```python
from build123d import *

# Parameters (mm, degrees)
SKETCH1_W           = 44.45
SKETCH1_H           = 50.8
BOSS_EXTRUDE1_DEPTH = 6.35
SKETCH2_W           = 5.08
SKETCH2_H           = 50.8
BOSS_EXTRUDE2_DEPTH = 25.4
SKETCH3_W           = 5.08
SKETCH3_H           = 50.8
BOSS_EXTRUDE3_DEPTH = 19.05
CUT_EXTRUDE1_REACH  = 55.295
CUT_EXTRUDE2_REACH  = 55.295
SKETCH5_R           = 1.905
LPATTERN1_COUNT     = 2
LPATTERN1_PITCH     = 12.7
LPATTERN1_COL_COUNT = 2
LPATTERN1_COL_PITCH = 12.7
CHAMFER3_SIZE       = 5.028946
CHAMFER1_SIZE       = 3.175
CUT_EXTRUDE3_REACH  = 40.756
SKETCH6_W           = 34.392108
SKETCH6_H           = 5.08
LPATTERN2_COUNT     = 2
LPATTERN2_PITCH     = 15.24
LPATTERN2_COL_COUNT = 2
LPATTERN2_COL_PITCH = 15.24
CHAMFER4_SIZE       = 1.27


with BuildPart() as part:
    # Sketch1 → Boss-Extrude1 (new body)
    with BuildSketch(Plane(origin=(0, 0, 0), x_dir=(1, 0, 0), z_dir=(0, 1, 0))):
        Rectangle(SKETCH1_W, SKETCH1_H)
    extrude(amount=BOSS_EXTRUDE1_DEPTH)

    # Sketch2 → Boss-Extrude2 (add)
    with BuildSketch(Plane(origin=(0, 0, 0), x_dir=(1, 0, 0), z_dir=(0, 1, 0))):
        with Locations((-19.685, 0)):
            Rectangle(SKETCH2_W, SKETCH2_H)
    extrude(amount=BOSS_EXTRUDE2_DEPTH)

    # Sketch3 → Boss-Extrude3 (add)
    with BuildSketch(Plane(origin=(0, 0, 0), x_dir=(1, 0, 0), z_dir=(0, 1, 0))):
        with Locations((19.685, 0)):
            Rectangle(SKETCH3_W, SKETCH3_H)
    extrude(amount=BOSS_EXTRUDE3_DEPTH)

    # Sketch4 → Cut-Extrude1 (cut, up to next)
    with BuildSketch(Plane(origin=(-17.145, 0, 0), x_dir=(0, 0, -1), z_dir=(1, 0, 0)), mode=Mode.PRIVATE) as cut_extrude1_sk1:
        with BuildLine():
            Line((-2.38125, 11.90625), (-2.38125, 19.84375))
            ThreePointArc((-2.38125, 19.84375), (0, 22.225), (2.38125, 19.84375))
            Line((2.38125, 19.84375), (2.38125, 11.90625))
            ThreePointArc((2.38125, 11.90625), (0, 9.525), (-2.38125, 11.90625))
        make_face()
    cut_extrude1_tool1 = extrude(cut_extrude1_sk1.sketch, amount=-CUT_EXTRUDE1_REACH, mode=Mode.PRIVATE) & part.part
    cut_extrude1 = cut_extrude1_tool1.solids().sort_by_distance((-17.145, 15.875, 0))[0]
    add(cut_extrude1, mode=Mode.SUBTRACT)

    # Sketch5 → Cut-Extrude2 (cut, up to next)
    with BuildSketch(Plane.ZY.offset(-17.145), mode=Mode.PRIVATE) as cut_extrude2_sk1:
        with Locations((0, 12.7)):
            Circle(SKETCH5_R)
    cut_extrude2_tool1 = extrude(cut_extrude2_sk1.sketch, amount=-CUT_EXTRUDE2_REACH, mode=Mode.PRIVATE) & part.part
    cut_extrude2 = cut_extrude2_tool1.solids().sort_by_distance((17.145, 12.7, 0))[0]
    add(cut_extrude2, mode=Mode.SUBTRACT)

    # LPattern1: Cut-Extrude1, Cut-Extrude2 ×2
    with Locations(*[(0, 0, i * LPATTERN1_PITCH) for i in range(1, LPATTERN1_COUNT)]):
        add(cut_extrude1, mode=Mode.SUBTRACT)
        add(cut_extrude2, mode=Mode.SUBTRACT)

    # LPattern1 col: Cut-Extrude1, Cut-Extrude2 ×2
    with Locations(*[(0, 0, -i * LPATTERN1_COL_PITCH) for i in range(1, LPATTERN1_COL_COUNT)]):
        add(cut_extrude1, mode=Mode.SUBTRACT)
        add(cut_extrude2, mode=Mode.SUBTRACT)

    # Chamfer3
    chamfer3_edges = [part.edges().sort_by_distance(p)[0] for p in [
        (22.225, 0, 0),
        (-22.225, 0, 0),
    ]]
    chamfer(chamfer3_edges, length=CHAMFER3_SIZE)

    # Chamfer1
    chamfer1_edges = [part.edges().sort_by_distance(p)[0] for p in [
        (-17.145, 15.875, 25.4),
        (-17.145, 15.875, -25.4),
        (-17.145, 25.4, 0),
        (17.145, 12.7, -25.4),
        (17.145, 12.7, 25.4),
        (17.145, 19.05, 0),
    ]]
    chamfer(chamfer1_edges, length=CHAMFER1_SIZE - 0.0001)  # a hair under: the kernel refuses the full size

    # Sketch6 → Cut-Extrude3 (cut, up to next)
    with BuildSketch(Plane(origin=(0, 6.35, 0), x_dir=(1, 0, 0), z_dir=(0, 1, 0)), mode=Mode.PRIVATE) as cut_extrude3_sk1:
        Rectangle(SKETCH6_W, SKETCH6_H)
    cut_extrude3_tool1 = extrude(cut_extrude3_sk1.sketch, amount=-CUT_EXTRUDE3_REACH, mode=Mode.PRIVATE) & part.part
    cut_extrude3 = cut_extrude3_tool1.solids().sort_by_distance((0, 6.35, 0))[0]
    add(cut_extrude3, mode=Mode.SUBTRACT)

    # LPattern2: Cut-Extrude3 ×2
    with Locations(*[(0, 0, i * LPATTERN2_PITCH) for i in range(1, LPATTERN2_COUNT)]):
        add(cut_extrude3, mode=Mode.SUBTRACT)

    # LPattern2 col: Cut-Extrude3 ×2
    with Locations(*[(0, 0, -i * LPATTERN2_COL_PITCH) for i in range(1, LPATTERN2_COL_COUNT)]):
        add(cut_extrude3, mode=Mode.SUBTRACT)

    # Chamfer4
    chamfer4_edges = [part.edges().sort_by_distance(p)[0] for p in [
        (0, 0, 25.4),
        (0, 0, -25.4),
        (17.145, 6.35, -20.00255),
        (-17.145, 6.35, 20.00255),
        (18.73245, 6.35, 23.81255),
        (-18.73245, 6.35, -23.81255),
        (17.145, 6.35, 7.62),
        (-17.145, 6.35, -7.62),
        (0, 0, 2.54),
        (0, 0, -2.54),
        (17.145, 6.35, -7.62),
        (-17.145, 6.35, -20.00255),
        (0, 0, -12.7),
        (0, 0, -17.78),
        (17.145, 6.35, 20.00255),
        (-17.145, 6.35, 7.62),
        (0, 0, 17.78),
        (0, 0, 12.7),
    ]]
    chamfer(chamfer4_edges, length=CHAMFER4_SIZE)


solid = part.part
```
The listing builds one solid part. Answer for the finished solid, in the listing's coordinates (mm). A direction names the side the tool comes from. Give positions to 0.01 mm unless a question says otherwise; leave off trailing zeros. Order: outer loops, then holes, each group sorted by start corner. A loop starts at its lowest first (then second) coordinate and runs counter-clockwise, first axis right, second up.
1) Consider line 1 along Z through (x, y) = (1.5, 5.5); line 2 along X through (y, z) = (15.25, -20) (3 decimals); line 3 along Y through (x, z) = (0, 20.5). Determine where each line is inside the solid, lowest interval first.
Reported:
line 1: z = -25.4 to -17.78, -12.7 to -2.54, 2.54 to 12.7, 17.78 to 25.4
line 2: x = -22.225 to -17.145, 17.145 to 22.225
line 3: y = 0 to 6.35
2) Find section A-A on z = -16.5. Write down the section's boundary in (x, y) (3 decimals).
Reported:
outline: (-22.225, 5.029) - (-17.196, 0) - (-17.196, 6.35) - (-17.145, 6.35) - (-17.145, 22.225) - (-20.32, 25.4) - (-22.225, 25.4) - close; (17.145, 6.35) - (17.196, 6.35) - (17.196, 0) - (22.225, 5.029) - (22.225, 19.05) - (20.32, 19.05) - (17.145, 15.875) - close
3) Find section D-D on y = 18. Write down the section's boundary in (x, z) (3 decimals).
Reported:
outline: (-22.225, -25.4) - (-20.32, -25.4) - (-17.145, -22.225) - (-17.145, -15.081) - (-22.225, -15.081) - close; (-22.225, -10.319) - (-17.145, -10.319) - (-17.145, -2.381) - (-22.225, -2.381) - close; (-22.225, 2.381) - (-17.145, 2.381) - (-17.145, 10.319) - (-22.225, 10.319) - close; (-22.225, 15.081) - (-17.145, 15.081) - (-17.145, 22.225) - (-20.32, 25.4) - (-22.225, 25.4) - close; (19.27, -24.35) - (20.32, -25.4) - (22.225, -25.4) - (22.225, 25.4) - (20.32, 25.4) - (19.27, 24.35) - close
4) For faces 1 (the face through (-20, 16, -2.381)), 2 (the face through (0, 6.35, 8)), 3 (the face through (17.196, 3, 0)), determine the directions among +Z, -Z, +X, -X, +Y, -Y from which every point of the face is accessible in a straight line to the end or side of a thin tool.
Reported:
face 1: -X
face 2: +Z, -Z, +Y
face 3: -Y
5) Given P1, Ø6, axis at y = 12.7, z = 12.7, coming from the +X side (3 decimals); P2, Ø1.5, axis at x = 5, z = -3, coming from the -Y side; P3, Ø1.5, axis at x = 17, y = 11, coming from the -Z side; P4, Ø3, axis at x = 17.5, z = 11.5, coming from the +Y side, each flat-ended and moving along its own axis, determine where each tip first touches the part or whether it passes through.
Reported:
P1: stops at x = 22.225
P2: stops at y = 0.06
P3: stops at z = -22.83
P4: stops at y = 17.73
6) Determine the mould class of faces 4 (the face through (-19.649, 22.224, 12.752)), 5 (the face through (-17.196, 3, 15)), 6 (the face through (16.519, 6.994, 20.231)) for opening direction Y: pulls with the +Y half, pulls with the -Y half, needs draft (parallel to the pull), parting line crosses it, or undercut.
Reported:
face 4: undercut
face 5: needs draft
face 6: pulls with the +Y half
7) Find section C-C on z = 0. Give the number of separate pieces and of enclosed holes in the cut face, then the cut area to 3 significant figures.
Reported:
separate pieces: 4
enclosed holes: 0
area: 106 mm2
8) Find section B-B on x = 7. Write down the section's boundary in (y, z).
Reported:
outline: (0, -24.13) - (1.27, -25.4) - (6.35, -25.4) - (6.35, -17.78) - (1.27, -17.78) - (0, -19.05) - close; (0, -11.43) - (1.27, -12.7) - (6.35, -12.7) - (6.35, -2.54) - (1.27, -2.54) - (0, -3.81) - close; (0, 3.81) - (1.27, 2.54) - (6.35, 2.54) - (6.35, 12.7) - (1.27, 12.7) - (0, 11.43) - close; (0, 19.05) - (1.27, 17.78) - (6.35, 17.78) - (6.35, 25.4) - (1.27, 25.4) - (0, 24.13) - close
